Check sheet for the modelled part. Datum: model origin and axes. Units: mm. A direction names the side the tool comes from. Give positions to 0.01 mm unless a question says otherwise; leave off trailing zeros. Order: outer loops, then holes, each group sorted by start corner. A loop starts at its lowest first (then second) coordinate and runs counter-clockwise, first axis right, second up.
Item 1: Release check for a two-part mould opening along Z. For faces 1 (the flat face through (1, 6, -10)), 2 (the flat face through (2.9, 21, -10)), 3 (the flat face through (10, 19, 0)) record: released by +Z, released by -Z, zero draft, split by the parting line, or undercut.
Item 2: Sectioned sample at C-C on x = 23.5. Record the boundary of the cut face in (y, z).
Item 3: Sectioned sample at D-D on y = 10. Record the boundary of the cut face in (x, z), and give its area (3 significant figures).
Item 4: Sectioned sample at B-B on z = -10.2. Record the boundary of the cut face in (x, y).
Item 5: Access from +Z, -Z, +X, -X, +Y, -Y to the whole of each face (thin tool, end or side, straight path). Record for faces 4 (the flat face through (9, 17, -3)), 5 (the cylindrical face through (24.1, 1.5, -10.2)), 6 (the flat face through (1, 30, -10)).
Item 6: Gauge pin test, flat ends, axial feed: P1, Ø6.5, axis at x = 11.19, y = 11.37, coming from the -Z side; P2, Ø6.5, axis at y = 26.5, z = -9, coming from the -X side; P3, Ø4, axis at x = 15, z = -7.5, coming from the +Y side; P4, Ø10, axis at x = 20, z = -16.5, coming from the +Y side. Record the tip position at first contact, or that the pin passes through.
Item 7: Material ranges on line 1 along Z through (x, y) = (2.85, 10); line 2 along Y through (x, z) = (6.4, -18.65); line 3 along Z through (x, y) = (11.5, 3), recorded low to high.
Item 8: Sectioned sample at A-A on y = 23.7. Record the boundary of the cut face in (x, z).
from build123d import *

# Parameters (mm, degrees)
CROQUIS1_R              = 5.59
CROQUIS1_R_2            = 1.6
SALIENTE_EXTRUIR1_DEPTH = 20.4
CROQUIS2_W              = 24.4
CROQUIS2_H              = 14.4
CORTAR_EXTRUIR1_DEPTH   = 35.1
CROQUIS3_R              = 1.5
CORTAR_EXTRUIR2_DEPTH   = 10
CORTAR_EXTRUIR3_DEPTH   = 10


with BuildPart() as part:
    # Croquis1 → Saliente-Extruir1 (new body)
    with BuildSketch(Plane.XY):
        Polygon((0, 0), (27.3, 0), (27.3, 2.9), (2.9, 38), (0, 38), (0, 30), (2.6, 30), (2.6, 22), (0, 22), (0, 14), (2.6, 14), (2.6, 6), (0, 6), align=None)
        with Locations((11.19, 11.3737)):
            Circle(CROQUIS1_R, mode=Mode.SUBTRACT)
        with Locations((6.4, 23.7)):
            Circle(CROQUIS1_R_2, mode=Mode.SUBTRACT)
    extrude(amount=-SALIENTE_EXTRUIR1_DEPTH)

    # Croquis2 → Cortar-Extruir1 (cut)
    with BuildSketch(Plane(origin=(0, 38, 0), x_dir=(1, 0, 0), z_dir=(0, 1, 0))):
        with Locations((15.1, 10.2)):
            Rectangle(CROQUIS2_W, CROQUIS2_H)
    extrude(amount=-CORTAR_EXTRUIR1_DEPTH, mode=Mode.SUBTRACT)

    # Croquis3 → Cortar-Extruir2 (cut)
    with BuildSketch(Plane.ZY.offset(-2.6)):
        with Locations(Location((-10.2, 26, 0), (0, 0, 270))):
            Circle(CROQUIS3_R)
        with Locations(Location((-10.2, 10, 0), (0, 0, 270))):
            Circle(CROQUIS3_R)
    extrude(amount=-CORTAR_EXTRUIR2_DEPTH, mode=Mode.SUBTRACT)

    # Croquis4 → Cortar-Extruir3 (cut)
    with BuildSketch(Plane(origin=(0, 2.9, 0), x_dir=(1, 0, 0), z_dir=(0, 1, 0))):
        with BuildLine():
            Line((22.6, 8.7), (7.6, 8.7))
            ThreePointArc((7.6, 8.7), (6.1, 10.2), (7.6, 11.7))
            Line((7.6, 11.7), (22.6, 11.7))
            ThreePointArc((22.6, 11.7), (24.1, 10.2), (22.6, 8.7))
        make_face()
    extrude(amount=-CORTAR_EXTRUIR3_DEPTH, mode=Mode.SUBTRACT)


solid = part.part
Report:
1. face 1: zero draft
1. face 2: undercut
1. face 3: released by +Z
2. outline: (0, -20.4) - (8.37, -20.4) - (8.37, -17.4) - (2.9, -17.4) - (2.9, -11.4) - (0, -11.4) - close; (0, -9) - (2.9, -9) - (2.9, -3) - (8.37, -3) - (8.37, 0) - (0, 0) - close
3. outline: (2.6, -20.4) - (5.77, -20.4) - (5.77, -17.4) - (2.9, -17.4) - (2.9, -11.7) - (2.6, -11.7) - close; (2.6, -8.7) - (2.9, -8.7) - (2.9, -3) - (5.77, -3) - (5.77, 0) - (2.6, 0) - close; (16.61, -20.4) - (22.36, -20.4) - (22.36, -17.4) - (16.61, -17.4) - close; (16.61, -3) - (22.36, -3) - (22.36, 0) - (16.61, 0) - close
3. area: 57.0 mm2
4. outline: (0, 0) - (6.1, 0) - (6.1, 2.9) - (2.9, 2.9) - (2.9, 8.5) - (2.6, 8.5) - (2.6, 6) - (0, 6) - close; (0, 14) - (2.6, 14) - (2.6, 11.5) - (2.9, 11.5) - (2.9, 24.5) - (2.6, 24.5) - (2.6, 22) - (0, 22) - close; (0, 30) - (2.6, 30) - (2.6, 27.5) - (2.9, 27.5) - (2.9, 38) - (0, 38) - close; (24.1, 0) - (27.3, 0) - (27.3, 2.9) - (24.1, 2.9) - close
5. face 4: +X, +Y
5. face 5: +Y, -Y
5. face 6: +Z, -Z, -X
6. P1: passes through
6. P2: stops at x = 2.6
6. P3: stops at y = 2.9
6. P4: stops at y = 20.48
7. line 1: z = -20.4 to -11.7, -8.7 to 0
7. line 2: y = 0 to 8.49, 14.26 to 22.1, 25.3 to 32.97
7. line 3: z = -20.4 to -17.4, -3 to 0
8. outline: (2.6, -20.4) - (4.8, -20.4) - (4.8, -17.4) - (2.9, -17.4) - (2.9, -3) - (4.8, -3) - (4.8, 0) - (2.6, 0) - close; (8, -20.4) - (12.84, -20.4) - (12.84, -17.4) - (8, -17.4) - close; (8, -3) - (12.84, -3) - (12.84, 0) - (8, 0) - close
